Source: CAD feature listing. Evaluate the final solid. Frame: model axes, mm. Face numbers are marked on the shaded views. Give positions to 0.01 mm unless a question says otherwise; leave off trailing zeros. Order: outer loops, then holes, each group sorted by start corner. A loop starts at its lowest first (then second) coordinate and runs counter-clockwise, first axis right, second up.
1) Section B-B, the plane y = -8. Return loops of the section in (x, z), plus the area to 3 significant figures.
2) Section A-A, the plane x = -16.5. Return loops of the section in (y, z), plus the area to 3 significant figures.
3) Draft query along Y for the marked faces 1, 2, 3 and 4. Return one class per face: released by +Y, released by -Y, zero draft, split by the parting line, or undercut.
4) Section D-D, the plane x = -48.5. Return loops of the section in (y, z), plus the area to 3 significant figures.
5) Material intervals for line 1 (Y direction, x = -9, z = 34); line 2 (Z direction, x = 2.5, y = 91); line 3 (Y direction, x = -1, z = 12), sorted ascending.
6) First-contact query: P1, Ø4, axis at y = 68.5, z = 11.5, coming from the -X side; P2, Ø4, axis at y = 26.5, z = 27, coming from the -X side; P3, Ø1.5, axis at y = 58.5, z = 31.5, coming from the -X side. Flat tips, straight axial feed; report the tip coordinate or a pass-through.
7) Section C-C, the plane x = -2. Return loops of the section in (y, z), plus the area to 3 significant figures.
Autodesk Inventor part; units mm, degrees
ref_plane "YZ Plane" through (0, 0, 0) normal (1, 0, 0) x (0, 1, 0)
ref_plane "XZ Plane" through (0, 0, 0) normal (0, 1, 0) x (-1, 0, 0)
ref_plane "XY Plane" through (0, 0, 0) normal (0, 0, 1) x (1, 0, 0)
sketch "Sketch1" plane through (0, 0, 0) normal (0, 0, 1) x (1, 0, 0)
  line L0 (9.4247, 103.8012) -> (9.4247, -95.1988)
  line L1 (9.4247, -95.1988) -> (-52.5753, -88.1988)
  line L2 (-52.5753, -88.1988) -> (-24.5753, 103.8012)
  line L3 (-24.5753, 103.8012) -> (9.4247, 103.8012)
  point P0 (0, 0)
  dimension "d0" = 199
  dimension "d1" = 62
  dimension "d2" = 34
  dimension "d3" = 7
extrude "Extrusion1" add sketch "Sketch1" along normal blind 39
sketch "Sketch2" plane through (9.4247, -95.1988, 0) normal (1, 0, 0) x (0, 0, -1)
  circle A0 centre (-11, 17) radius 4
  circle A1 centre (-25, 17) radius 4
  circle A2 centre (-15, 189) radius 4
  circle A3 centre (-29, 189) radius 4
  line L0 (-39, 0) -> (-39, 199)
  line L1 (0, 0) -> (-39, 0)
  line L2 (0, 199) -> (-39, 199)
  point P0 (0, 95.1988)
  dimension "d6" = 8
  dimension "d7" = 8
  dimension "d8" = 14
  dimension "d9" = 14
  dimension "d10" = 172
  dimension "d11" = 8
  dimension "d12" = 8
  dimension "d13" = 14
  dimension "d14" = 10
  dimension "d18" = 10
extrude "Extrusion2" cut sketch "Sketch2" against normal through all
sketch "Sketch3" plane through (0, 0, 39) normal (0, 0, 1) x (1, 0, 0)
  circle A0 centre (-16.0753, -11.3988) radius 9
  circle A1 centre (-11.5753, 34.8012) radius 7.5
  line L0 (9.4247, -95.1988) -> (9.4247, 103.8012)
  line L1 (9.4247, 103.8012) -> (-24.5753, 103.8012)
  point P0 (0, 0)
  dimension "d19" = 18
  dimension "d20" = 15
  dimension "d21" = 25.5
  dimension "d22" = 21
  dimension "d23" = 69
  dimension "d24" = 115.2
extrude "Extrusion3" cut sketch "Sketch3" against normal through all
properties part number "Ball screw support [bed]"
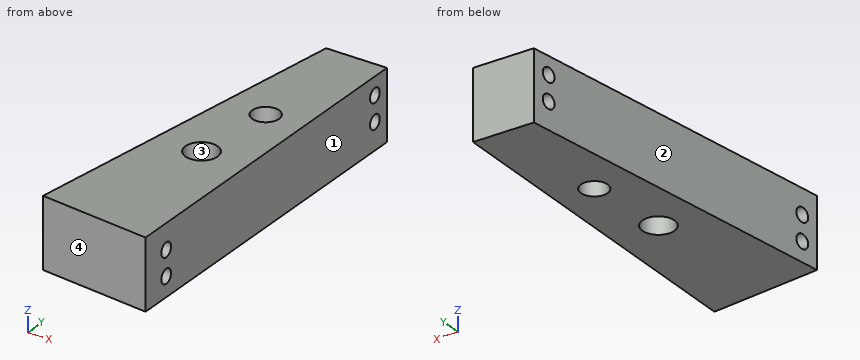
From the geometry:
1. outline: (-40.88, 0) - (-24.41, 0) - (-24.41, 39) - (-40.88, 39) - close; (-7.74, 0) - (9.42, 0) - (9.42, 39) - (-7.74, 39) - close
1. area: 1,310 mm2
2. outline: (-92.27, 0) - (-20.39, 0) - (-20.39, 39) - (-92.27, 39) - close; (-2.41, 0) - (29.14, 0) - (29.14, 39) - (-2.41, 39) - close; (40.46, 0) - (103.8, 0) - (103.8, 39) - (40.46, 39) - close; hole circle Ø8 at (-78.2, 11); hole circle Ø8 at (-78.2, 25); hole circle Ø8 at (93.8, 15); hole circle Ø8 at (93.8, 29)
2. area: 6,300 mm2
3. face 1: zero draft
3. face 2: released by +Y
3. face 3: undercut
3. face 4: released by -Y
4. outline: (-88.66, 0) - (-60.25, 0) - (-60.25, 39) - (-88.66, 39) - close; hole circle Ø8 at (-78.2, 11); hole circle Ø8 at (-78.2, 25)
4. area: 1,010 mm2
5. line 1: y = -93.12 to -16.96, -5.84 to 27.76, 41.85 to 103.8
5. line 2: z = 0 to 12.14, 17.86 to 26.14, 31.86 to 39
5. line 3: y = -94.02 to -82.07, -74.33 to 91.16, 96.45 to 103.8
6. P1: stops at x = -30.02
6. P2: stops at x = -36.14
6. P3: stops at x = -31.29
7. outline: (-93.91, 0) - (103.8, 0) - (103.8, 39) - (-93.91, 39) - close; hole circle Ø8 at (-78.2, 11); hole circle Ø8 at (-78.2, 25); hole circle Ø8 at (93.8, 15); hole circle Ø8 at (93.8, 29)
7. area: 7,510 mm2
